Design review of the part built by this model. Coordinates are the model's own, in mm. Face numbers are marked on the shaded views. A direction names the side the tool comes from. Coordinates: 2 decimals unless noted, no trailing zeros. Write each loop counter-clockwise with the first axis right and the second up, starting at its lowest first coordinate (ties: lowest second). Pieces come first, ordered by that corner, then holes. Notation, with made-up numbers: (-16, -19.75) - (-7, -19.75) arc R28 cw to (-7, 19.25) - close; hole circle Ø3 at (16, 3.5). An arc over 180 degrees is marked (long way). Answer as a JSON object with one key per item and string values.
Autodesk Inventor part; units mm, degrees
ref_plane "YZ Plane" through (0, 0, 0) normal (1, 0, 0) x (0, 1, 0)
ref_plane "XZ Plane" through (0, 0, 0) normal (0, 1, 0) x (-1, 0, 0)
ref_plane "XY Plane" through (0, 0, 0) normal (0, 0, 1) x (1, 0, 0)
sketch "Sketch1" plane through (0, 0, 0) normal (0, 1, 0) x (-1, 0, 0)
  circle A0 centre (0, 0) radius 7
  circle A1 centre (0, 0) radius 8 construction
  line L0 (0, 0) -> (5.6569, -5.6569) construction
  line L1 (0, 0) -> (8, 0) construction
  line L2 (0, 0) -> (-5.6569, -5.6569) construction
  line L3 (0, 0) -> (8, 0) construction
  line L4 (0, 0) -> (5.6569, 5.6569) construction
  line L5 (0, 0) -> (-5.6569, 5.6569) construction
  arc A2 (5.6319, 4.1571) -> (4.1571, 5.6319) centre (5.6569, 5.6569) ccw
  arc A3 (-4.1571, 5.6319) -> (-5.6319, 4.1571) centre (-5.6569, 5.6569) ccw
  arc A4 (-5.6319, -4.1571) -> (-4.1571, -5.6319) centre (-5.6569, -5.6569) ccw
  arc A5 (4.1571, -5.6319) -> (5.6319, -4.1571) centre (5.6569, -5.6569) ccw
  arc A6 (4.5962, 4.5962) -> (5.6319, 4.1571) centre (5.6569, 5.6569) ccw
  arc A7 (4.1571, 5.6319) -> (4.5962, 4.5962) centre (5.6569, 5.6569) ccw
  arc A8 (-4.5962, 4.5962) -> (-4.1571, 5.6319) centre (-5.6569, 5.6569) ccw
  arc A9 (-5.6319, 4.1571) -> (-4.5962, 4.5962) centre (-5.6569, 5.6569) ccw
  arc A10 (-4.5962, -4.5962) -> (-5.6319, -4.1571) centre (-5.6569, -5.6569) ccw
  arc A11 (-4.1571, -5.6319) -> (-4.5962, -4.5962) centre (-5.6569, -5.6569) ccw
  arc A12 (4.5962, -4.5962) -> (4.1571, -5.6319) centre (5.6569, -5.6569) ccw
  arc A13 (5.6319, -4.1571) -> (4.5962, -4.5962) centre (5.6569, -5.6569) ccw
  line L6 (-20, 7.25) -> (20, 7.25)
  line L7 (20, 7.25) -> (20, -7.25) construction
  line L8 (20, -7.25) -> (-20, -7.25) construction
  line L9 (-20, -7.25) -> (-20, 7.25) construction
  line L10 (-20, 7.25) -> (20, -7.25) construction
  line L11 (20, 7.25) -> (-20, -7.25) construction
  line L12 (20, 7.25) -> (-20, 7.25)
  line L13 (-20, 7.25) -> (-20, 27.25)
  line L14 (-20, 27.25) -> (20, 27.25)
  line L15 (20, 27.25) -> (20, 7.25)
  line L16 (20, 17.25) -> (-20, 17.25) construction
  circle A14 centre (10, 17.25) radius 2.5
  circle A15 centre (-10, 17.25) radius 2.5
  line L17 (20, 7.25) -> (-20, 7.25)
  line L18 (-20, 7.25) -> (-20, -10.75)
  line L19 (-20, -10.75) -> (20, -10.75)
  line L20 (20, -10.75) -> (20, 7.25)
  dimension "d0" = 14
  dimension "d1" = 16
  dimension "d2" = 45
  dimension "d3" = 135
  dimension "d4" = 3
  dimension "d5" = 3
  dimension "d6" = 3
  dimension "d7" = 3
  dimension "d9" = 14.5
  dimension "d10" = 20
  dimension "d11" = 40
  dimension "d14" = 5
  dimension "d15" = 5
  dimension "d16" = 10
  dimension "d17" = 10
  dimension "d22" = 18
  dimension "d23" = 40
  dimension "d24" = 40
extrude "Extrusion1" add sketch "Sketch1" along normal blind 5 contours L13 L14 L15 L6
extrude "Extrusion3" add sketch "Sketch1" along normal blind 25 contours L6 L20 L19 L18
sketch "Sketch3" plane through (0, 25, 0) normal (0, 1, 0) x (1, 0, 0)
  line L0 (20, -27.25) -> (20, -7.25)
  line L1 (-20, 10.75) -> (20, 10.75)
  line L2 (20, 10.75) -> (20, -27.25)
  line L3 (20, -27.25) -> (-20, -27.25)
  line L4 (-20, -27.25) -> (-20, 10.75)
  point P0 (0, 0)
extrude "Extrusion4" add sketch "Sketch3" along normal blind 5
extrude "Extrusion5" cut sketch "Sketch1" along normal blind 30 contours A0 A13 A12 A11 A10 A9 A8 A7 A6 | A6 A7 A0 | A0 A2 | A5 A0 | A0 A12 A13 | A8 A9 A0 | A0 A3 | A4 A0 | A0 A10 A11 | A14 | A15
fillet "Fillet2" radius 1 24 edges at (-20, 15, 7.25) (0, 25, 7.25) (-20, 25, 17.25) (0, 25, 27.25) (-20, 27.5, 27.25) (0, 30, 27.25) (20, 27.5, 27.25) (20, 25, 17.25) (-20, 30, 8.25) (-20, 15, -10.75) (-20, 5, 17.25) (-20, 2.5, 27.25) (0, 5, 27.25) (0, 0, 27.25) (-20, 0, 8.25) (20, 0, 8.25) (20, 2.5, 27.25) (20, 15, 7.25) (0, 5, 7.25) (20, 5, 17.25) (20, 30, 8.25) (20, 15, -10.75) (0, 30, -10.75) (0, 0, -10.75)
equation "\"d4\" = d5"
equation "\"d6\" = d5"
equation "\"d7\" = d5"
equation "\"d11\" = d13"
equation "\"d17\" = d16"
equation "\"d24\" = d23"
properties part number "z_nut_holder" material "ABS Plastic"
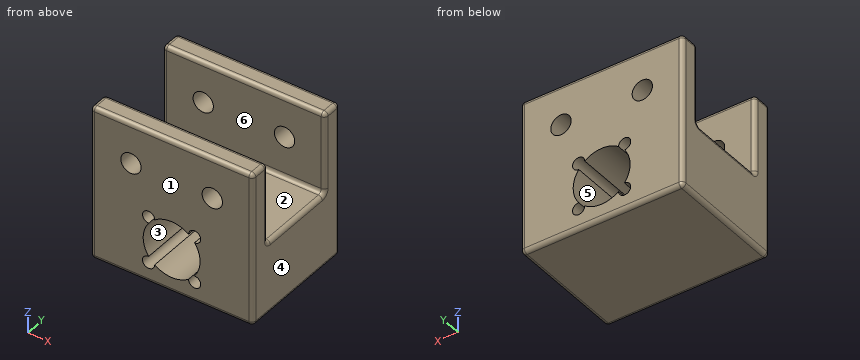
(1) Take a section at C-C, the plane y = 27. Write out the cut boundary in (x, z).
Solved:
{"outline": "(-20, -9.75) arc R1 ccw to (-19, -10.75) - (19, -10.75) arc R1 ccw to (20, -9.75) - (20, 26.25) arc R1 ccw to (19, 27.25) - (-19, 27.25) arc R1 ccw to (-20, 26.25) - close; hole circle Ø5 at (-10, 17.25); hole (-5.63, -4.16) arc R1.5 ccw (long way) to (-4.16, -5.63) arc R7 ccw to (4.16, -5.63) arc R1.5 ccw (long way) to (5.63, -4.16) arc R7 ccw to (5.63, 4.16) arc R1.5 ccw (long way) to (4.16, 5.63) arc R7 ccw to (-4.16, 5.63) arc R1.5 ccw (long way) to (-5.63, 4.16) arc R7 ccw to start; hole circle Ø5 at (10, 17.25)"}
(2) For pin 1 (4 mm diameter, centred on x = 6, y = 16.5, fed in from +Z), flat-tipped, find the tip position at first contact; note if it passes through.
Solved:
{"pin 1": "stops at z = 7.25"}
(3) Take a section at A-A, the plane z = 17.25. Give the number of separate pieces and of enclosed holes in the cut face, and give its area (3 significant figures).
Solved:
{"separate pieces": "6", "enclosed holes": "0", "area": "298 mm^2"}
(4) Take a section at D-D, the plane z = -3. Write out the cut boundary in (x, y).
Solved:
{"outline": "(-20, 1) arc R1 ccw to (-19, 0) - (-6.32, 0) - (-6.32, 30) - (-19, 30) arc R1 ccw to (-20, 29) - close; (6.32, 0) - (19, 0) arc R1 ccw to (20, 1) - (20, 29) arc R1 ccw to (19, 30) - (6.32, 30) - close"}
(5) Take a section at B-B, the plane x = -10. Write out the cut boundary in (y, z).
Solved:
{"outline": "(0, -9.75) arc R1 ccw to (1, -10.75) - (29, -10.75) arc R1 ccw to (30, -9.75) - (30, 14.75) - (25, 14.75) - (25, 8.25) arc R1 cw to (24, 7.25) - (6, 7.25) arc R1 cw to (5, 8.25) - (5, 14.75) - (0, 14.75) - close; (0, 19.75) - (5, 19.75) - (5, 26.25) arc R1 ccw to (4, 27.25) - (1, 27.25) arc R1 ccw to (0, 26.25) - close; (25, 19.75) - (30, 19.75) - (30, 26.25) arc R1 ccw to (29, 27.25) - (26, 27.25) arc R1 ccw to (25, 26.25) - close"}
(6) To check wall thickness, follow line 1 (X direction, y = 28.25, z = 17.25); line 2 (Y direction, x = 3.5, z = 14); line 3 (Z direction, x = -5, y = 11.75). State the ranges of each line that lie inside material, in increasing order. Write a range as from..to.
Solved:
{"line 1": "x = -20..-12.5, -7.5..7.5, 12.5..20", "line 2": "y = 0..5, 25..30", "line 3": "z = -10.75..-7.01, 7.01..7.25"}
(7) The part is to be moulded in two halves that separate along X. For the marked faces 4, 5 and 6, say which applies: pulls with the +X half, pulls with the -X half, needs draft (parallel to the pull), parting line crosses it, or undercut.
Solved:
{"face 4": "pulls with the +X half", "face 5": "undercut", "face 6": "needs draft"}
(8) Tool access review of the marked faces 1, 2 and 3: name each direction out of +Z, -Z, +X, -X, +Y, -Y from which nothing blocks a thin tool from reaching the whole face with its end or side.
Solved:
{"face 1": "+Z, -Z, +X, -X, -Y", "face 2": "+Z, +X, -X", "face 3": "+Y, -Y"}
